For this review, take the finished solid that the model builds, in its own axes (mm). A direction names the side the tool comes from. Coordinates: 2 decimals unless noted, no trailing zeros. Write each loop counter-clockwise with the first axis right and the second up, starting at its lowest first coordinate (ties: lowest second). Pieces come first, ordered by that corner, then holes. Notation, with made-up numbers: (18.5, -0.75) -> (71.5, -0.75) arc R15 ccw to (71.5, 8.25) -> close; hole circle Ø11 at (4, 70.25). An arc over 180 degrees is marked (long way). Put each result on its own line as item: value. Start each with the question number.
Item 1: Insertion check: P1, Ø15, axis at x = -43.5, z = 12, coming from the +Y side; P2, Ø18, axis at x = -74.94, y = 40, coming from the -Z side; P3, Ø4, axis at x = -77.5, z = -14.5, coming from the +Y side; P4, Ø13, axis at y = 30, z = 18.5, coming from the +X side. Each pin has a flat end and moves straight along its axis. Give the tip position at first contact, or say it passes through.
Item 2: The part is to be moulded in two halves that separate along Z. For faces 4 (the flat face through (-57, 23, 25)), 5 (the cylindrical face through (-89.297, 53.986, -19.084)), 6 (the cylindrical face through (-2.17, 9.86, -9.76)), say which applies: +Z half, -Z half, draft (parallel to the pull), parting line (faces both ways), or undercut.
Item 3: Consider section B-B on y = 42. Give the boundary of the cut face in (x, z), and give its area (3 significant figures).
Item 4: Consider section A-A on z = 0. Give the boundary of the cut face in (x, y), and give its area (3 significant figures).
Item 5: To check wall thickness, follow L1, parallel to Z at x = 0, y = 12; L2, parallel to Z at x = -85.5, y = 40; L3, parallel to Y at x = -76.5, z = 11.5. State the ranges of each line that lie inside material, in increasing order.
Item 6: For faces 1 (the flat face through (-70, 31, -13)), 2 (the flat face through (-59, 23, -25)), 3 (the flat face through (-55, 30, -19)), list the 3-axis set-ups (+Z, -Z, +X, -X, +Y, -Y) from which the entire face can be reached by the end or side of a thin tool; tool diameter is ignored.
Item 7: Consider section D-D on x = -58.5. Give the boundary of the cut face in (y, z).
Solid Edge part; units mm, degrees
sketch "Sketch1" plane through (0, 0, 0) normal (0, -1, 0) x (1, 0, 0)
  line L0 (-55, -25) -> (0, -25)
  line L1 (-55, -13) -> (-55, -25)
  line L2 (-95, -13) -> (-55, -13)
  line L3 (-95, 13) -> (-95, -13)
  line L4 (-55, 13) -> (-95, 13)
  line L5 (-55, 25) -> (-55, 13)
  line L6 (0, 25) -> (-55, 25)
  arc A0 (0, 25) -> (0, -25) centre (0, 0) cw
  circle A1 centre (0, 0) radius 10
extrude "Protrusion1" add sketch "Sketch1" against normal blind 20
sketch "Sketch2" plane through (0, 0, 0) normal (0, -1, 0) x (1, 0, 0)
  line L0 (-95, -25) -> (-55, -25)
  line L1 (-55, -25) -> (-55, -13)
  line L2 (-55, -13) -> (-95, -13)
  line L3 (-95, -13) -> (-95, -25)
  line L4 (-95, 13) -> (-55, 13)
  line L5 (-55, 13) -> (-55, 25)
  line L6 (-55, 25) -> (-95, 25)
  line L7 (-95, 25) -> (-95, 13)
extrude "ExtrudedProtrusion_5" add sketch "Sketch2" against normal blind 60
fillet "Round_2" radius 20 4 edges at (-55, 60, -19) (-95, 60, -19) (-55, 60, 19) (-95, 60, 19)
sketch "Sketch3" plane through (-47.5, 30, -25) normal (0, 0, -1) x (-1, 0, 0)
  circle A0 centre (27.4446, 10) radius 10
extrude "ExtrudedCutout_1" cut sketch "Sketch3" against normal blind 50
Return value:
1. P1: y = 20
1. P2: through
1. P3: y = 59.99
1. P4: x = -55
2. face 4: +Z half
2. face 5: draft
2. face 6: undercut
3. outline: (-94.9, -25) -> (-84.74, -25) -> (-84.74, -13) -> (-94.9, -13) -> close; (-94.9, 13) -> (-84.74, 13) -> (-84.74, 25) -> (-94.9, 25) -> close; (-65.15, -25) -> (-55.1, -25) -> (-55.1, -13) -> (-65.15, -13) -> close; (-65.15, 13) -> (-55.1, 13) -> (-55.1, 25) -> (-65.15, 25) -> close
3. area: 485 mm^2
4. outline: (-95, 0) -> (-10, 0) -> (-10, 20) -> (-95, 20) -> close; (10, 0) -> (25, 0) -> (25, 20) -> (10, 20) -> close
4. area: 2,000 mm^2
5. L1: -25 to -10, 10 to 25
5. L2: -25 to -13, 13 to 25
5. L3: 0 to 20
6. face 1: +X, -X, +Y
6. face 2: -Z, +X, -X, +Y, -Y
6. face 3: +Z, -Z, +X, +Y
7. outline: (0, -25) -> (51.3, -25) -> (51.3, -13) -> (20, -13) -> (20, 13) -> (51.3, 13) -> (51.3, 25) -> (0, 25) -> close
